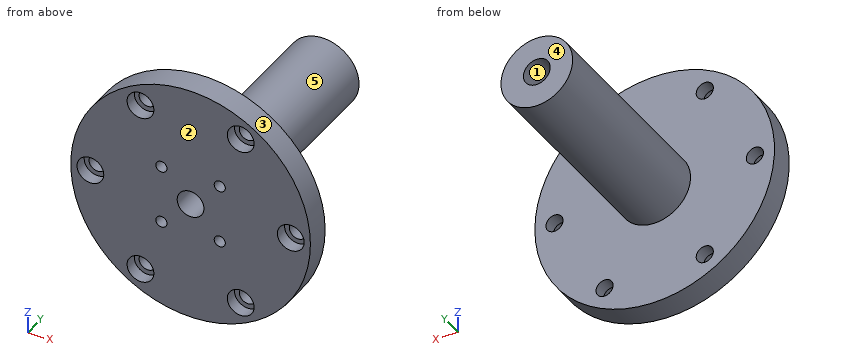
Autodesk Inventor part; units mm, degrees
ref_plane "YZ Plane" through (0, 0, 0) normal (1, 0, 0) x (0, 1, 0)
ref_plane "XZ Plane" through (0, 0, 0) normal (0, 1, 0) x (-1, 0, 0)
ref_plane "XY Plane" through (0, 0, 0) normal (0, 0, 1) x (1, 0, 0)
sketch "Sketch1" plane through (0, 0, 0) normal (0, 0, 1) x (1, 0, 0)
  line L0 (0, 0) -> (0, 26.4) construction
  line L1 (3.175, 0) -> (28.4, 0)
  line L2 (8.5, 6) -> (28.4, 6)
  line L3 (8.5, 53.9934) -> (8.5, 6)
  line L4 (28.4, 6) -> (28.4, 0)
  line L5 (3.175, 53.9934) -> (8.5, 53.9934)
  line L6 (3.175, 53.9934) -> (3.175, 0)
  dimension "d0" = 26.4
  dimension "d53" = 47.9934
revolve "Revolution1" add sketch "Sketch1" angle 360 about axis through (0, 0, 0) along (0, 1, 0)
sketch "Sketch5" plane through (0, 0, 0) normal (0, -1, 0) x (1, 0, 0)
  circle A0 centre (0, 0) radius 3.175
  line L0 (0, 0) -> (6.9148, -6.9148)
  line L1 (0, 0) -> (9.779, 0) construction
  dimension "d39" = 9.779
  dimension "d40" = 45
hole "Hole2" at (6.9148, 0, -6.9148) direction (0, 1, 0) diameter 2.6416 depth 5.08 tip angle 118
pattern_circular "Circular Pattern2" count 4 over 360 about axis through (0, 26.9967, 0) along (0, -1, 0) of "Hole2"
sketch "Sketch6" plane through (0, 0, 0) normal (0, -1, 0) x (1, 0, 0)
  point P0 (0, 0)
sketch "Sketch7" plane through (0, 0, 0) normal (0, -1, 0) x (1, 0, 0)
  line L0 (0, 0) -> (-23.749, 0) construction
  dimension "d57" = 23.749
hole "Hole3" at (-23.749, 0, 0) direction (0, 1, 0) diameter 4.064 end through all counterbore diameter 6.35 counterbore depth 2.921
pattern_circular "Circular Pattern3" count 6 over 360 about axis through (0, 26.9967, 0) along (0, -1, 0) of "Hole3"
properties part number "Mechanum Wheel Adapter"
Could you check a few things on this model? Use its own coordinates, in mm. Face numbers are marked on the shaded views. A direction names the side the tool comes from. Coordinates: 2 decimals unless noted, no trailing zeros. Write each loop counter-clockwise with the first axis right and the second up, starting at its lowest first coordinate (ties: lowest second). Pieces come first, ordered by that corner, then holes. Notation, with made-up numbers: M 16,40.5 L 68,40.5 A25 cw 68,58.5 Z; hole C 3.5,-33.5 d3. An arc over 180 degrees is marked long. Answer as CSV lines item,"result". Start each with the question number.
1) We'd pull the mould along X, two halves only. Please class the marked faces 1, 2 and 3: +X half, -X half, draft (parallel to the pull), parting line (faces both ways), or undercut.
2) For the marked faces 4 and 5, which set-ups out of +Z, -Z, +X, -X, +Y, -Y let a thin tool reach every point of the face, with its end or its side?
3) I want a section at D-D, the plane z = -13. Please give me the cut outline in (x, y), and give its area (3 significant figures).
4) I want a section at C-C, the plane y = 45. Please give me the cut outline in (x, z) (3 decimals), and give its area (3 significant figures).
5) For P1, Ø12, axis at x = 21.5, z = 19, coming from the +Y side; P2, Ø6, axis at x = -13.5, y = 28.5, coming from the +Z side; P3, Ø5, axis at y = 40.5, z = 8.5, coming from the -X side; P4, Ø12, axis at x = 5.5, y = 21.5, coming from the +Z side, each with a flat end and sliding along its axis, tell me the tip position at first contact or that it passes through.
6) Please list where these lines run through material, in increasing order: line 1 (Z direction, x = -7, y = 5); line 2 (Y direction, x = 21, z = 1); line 3 (Y direction, x = -22, z = -15.5). Write a range as from..to.
7) I want a section at B-B, the plane x = 0. Please give me the cut outline in (y, z) (3 decimals), and give its area (3 significant figures).
8) I want a section at A-A, the plane z = 0. Please give me the cut outline in (x, y) (3 decimals), and give its area (3 significant figures).
Data:
1,face 1,"undercut"
1,face 2,"draft"
1,face 3,"parting line"
2,face 4,"+Z, -Z, +X, -X, +Y"
2,face 5,"+Y"
3,outline,"M -25.25,0 L 25.25,0 L 25.25,6 L -25.25,6 Z"
3,area,"303 mm^2"
4,outline,"C 0,0 d17; hole C 0,0 d6.35"
4,area,"195 mm^2"
5,P1,"stops at y = 6"
5,P2,"passes through"
5,P3,"stops at x = -6.02"
5,P4,"stops at z = 8.5"
6,line 1,"z = -27.52..-8.23, -5.6..5.6, 8.23..27.52"
6,line 2,"y = 2.92..6"
6,line 3,"y = 0..6"
7,outline,"M 0,-28.4 L 6,-28.4 L 6,-8.5 L 53.993,-8.5 L 53.993,-3.175 L 0,-3.175 Z; M 0,3.175 L 53.993,3.175 L 53.993,8.5 L 6,8.5 L 6,28.4 L 0,28.4 Z"
7,area,"814 mm^2"
8,outline,"M -28.4,0 L -26.924,0 L -26.924,2.921 L -25.781,2.921 L -25.781,6 L -28.4,6 Z; M -21.717,2.921 L -20.574,2.921 L -20.574,0 L -3.175,0 L -3.175,53.993 L -8.5,53.993 L -8.5,6 L -21.717,6 Z; M 3.175,0 L 20.574,0 L 20.574,2.921 L 21.717,2.921 L 21.717,6 L 8.5,6 L 8.5,53.993 L 3.175,53.993 Z; M 25.781,2.921 L 26.924,2.921 L 26.924,0 L 28.4,0 L 28.4,6 L 25.781,6 Z"
8,area,"752 mm^2"
